The listing builds one solid part. Answer for the finished solid, in the listing's coordinates (mm). A direction names the side the tool comes from. Give positions to 0.01 mm unless a question says otherwise; leave off trailing zeros. Loops run counter-clockwise (first coordinate to the right, second up) from the corner with the lowest first, then second, coordinate; pieces in that order, holes last. Notation, with made-up numbers: (6, -34) - (15, -34) arc R23 ccw to (15, -23) - close; hole circle Ø1 at (-11, 2.25). An arc over 180 degrees is marked (long way). Write each question's results on one line, items separated by ' | '.
from build123d import *

# Parameters (mm, degrees)
SKETCH1_W           = 399.143716184
SKETCH1_H           = 508
SKETCH1_R           = 10
BOSS_EXTRUDE1_DEPTH = 20
SKETCH1_2_R         = 10
BOSS_EXTRUDE2_DEPTH = 60


with BuildPart() as part:
    # Sketch1 → Boss-Extrude1 (new body)
    with BuildSketch(Plane.XY):
        Rectangle(SKETCH1_W, SKETCH1_H)
        Circle(SKETCH1_R, mode=Mode.SUBTRACT)
        with Locations((0, 200)):
            Circle(SKETCH1_R, mode=Mode.SUBTRACT)
    extrude(amount=BOSS_EXTRUDE1_DEPTH)

    # Sketch1<2> → Boss-Extrude2 (add)
    with BuildSketch(Plane.XY):
        with Locations((0, 200)):
            Circle(SKETCH1_2_R)
    extrude(amount=BOSS_EXTRUDE2_DEPTH)


solid = part.part
Item 1: Find the intervals of material crossed by line 1 along Y through (x, z) = (0, 8.5); line 2 along Z through (x, y) = (-152, 57), in increasing order. Write a range as [from, to].
Values found:
line 1: y = [-254, -10], [10, 254] | line 2: z = [0, 20]
Item 2: A flat-ended cylindrical pin translates along its axis: P1, Ø2, axis at x = 152.5, y = -49.5, coming from the +Z side. Find the tip coordinate at first contact, or state that the pin passes through.
Values found:
P1: stops at z = 20
Item 3: A cutting plane is placed at B-B, the plane x = 0. Determine the outline of the cut face in (y, z).
Values found:
outline: (-254, 0) - (-10, 0) - (-10, 20) - (-254, 20) - close; (10, 0) - (254, 0) - (254, 20) - (210, 20) - (210, 60) - (190, 60) - (190, 20) - (10, 20) - close
Item 4: A cutting plane is placed at A-A, the plane y = 0. Determine the outline of the cut face in (x, z), plus the area to 3 significant figures.
Values found:
outline: (-199.57, 0) - (-10, 0) - (-10, 20) - (-199.57, 20) - close; (10, 0) - (199.57, 0) - (199.57, 20) - (10, 20) - close | area: 7,580 mm²
Item 5: For faces 4 (the face through (-199.572, -4, 10)), 5 (the face through (-2.17, 190.24, 39.72)), determine the directions among +Z, -Z, +X, -X, +Y, -Y from which every point of the face is accessible in a straight line to the end or side of a thin tool.
Values found:
face 4: +Z, -Z, -X, +Y, -Y | face 5: +Z
Item 6: A cutting plane is placed at D-D, the plane z = 32.5. Determine the outline of the cut face in (x, y).
Values found:
outline: circle Ø20 at (0, 200)
Item 7: A cutting plane is placed at C-C, the plane y = 200. Determine the outline of the cut face in (x, z).
Values found:
outline: (-199.57, 0) - (199.57, 0) - (199.57, 20) - (10, 20) - (10, 60) - (-10, 60) - (-10, 20) - (-199.57, 20) - close
Item 8: For a pull along X with two mould halves and no side action, classify faces 1 (the face through (-2.17, -9.76, 9.86)), 2 (the face through (0, 200, 60)), 3 (the face through (199.572, -4, 10)) as released by +X, released by -X, zero draft, split by the parting line, or undercut.
Values found:
face 1: undercut | face 2: zero draft | face 3: released by +X
